```python
from build123d import *

# Parameters (mm, degrees)
SKETCH1_R           = 13.335
SKETCH1_R_2         = 8.255
SKETCH1_R_3         = 1.8288
BOSS_EXTRUDE1_DEPTH = 0.762
BOSS_EXTRUDE2_START = 1.524
SKETCH2_R           = 13.335
SKETCH2_R_2         = 12.573
BOSS_EXTRUDE2_DEPTH = 1.524


with BuildPart() as part:
    # Sketch1 → Boss-Extrude1 (new body)
    with BuildSketch(Plane.XY):
        with Locations(Location((0, 0, 0), (0, 0, 180))):
            Circle(SKETCH1_R)
        with Locations(Location((0, 0, 0), (0, 0, 180))):
            Circle(SKETCH1_R_2, mode=Mode.SUBTRACT)
        with Locations(Location((8.919971224, 5.542595082, 0), (0, 0, 180))):
            Circle(SKETCH1_R_3, mode=Mode.SUBTRACT)
        with Locations(Location((10.496219222, 0.340042532, 0), (0, 0, 180))):
            Circle(SKETCH1_R_3, mode=Mode.SUBTRACT)
        with Locations(Location((9.260013756, -4.95362414, 0), (0, 0, 180))):
            Circle(SKETCH1_R_3, mode=Mode.SUBTRACT)
        with Locations(Location((5.542595082, -8.919971224, 0), (0, 0, 180))):
            Circle(SKETCH1_R_3, mode=Mode.SUBTRACT)
        with Locations(Location((0.340042532, -10.496219222, 0), (0, 0, 180))):
            Circle(SKETCH1_R_3, mode=Mode.SUBTRACT)
        with Locations(Location((-4.95362414, -9.260013756, 0), (0, 0, 180))):
            Circle(SKETCH1_R_3, mode=Mode.SUBTRACT)
        with Locations(Location((-8.919971224, -5.542595082, 0), (0, 0, 180))):
            Circle(SKETCH1_R_3, mode=Mode.SUBTRACT)
        with Locations(Location((-10.496219222, -0.340042532, 0), (0, 0, 180))):
            Circle(SKETCH1_R_3, mode=Mode.SUBTRACT)
        with Locations(Location((-9.260013756, 4.95362414, 0), (0, 0, 180))):
            Circle(SKETCH1_R_3, mode=Mode.SUBTRACT)
        with Locations(Location((-5.542595082, 8.919971224, 0), (0, 0, 180))):
            Circle(SKETCH1_R_3, mode=Mode.SUBTRACT)
        with Locations(Location((-0.340042532, 10.496219222, 0), (0, 0, 180))):
            Circle(SKETCH1_R_3, mode=Mode.SUBTRACT)
        with Locations(Location((4.95362414, 9.260013756, 0), (0, 0, 180))):
            Circle(SKETCH1_R_3, mode=Mode.SUBTRACT)
    extrude(amount=BOSS_EXTRUDE1_DEPTH)

    # Sketch2 → Boss-Extrude2 (add)
    with BuildSketch(Plane(origin=(0, 0, 0), x_dir=(-1, 0, 0), z_dir=(0, 0, -1)).offset(BOSS_EXTRUDE2_START)):
        Circle(SKETCH2_R)
        with Locations(Location((0, 0, 0), (0, 0, 180))):
            Circle(SKETCH2_R_2, mode=Mode.SUBTRACT)
    extrude(amount=-BOSS_EXTRUDE2_DEPTH)


solid = part.part
```
Check sheet for the modelled part. Datum: model origin and axes. Units: mm. A direction names the side the tool comes from. Coordinates: 2 decimals unless noted, no trailing zeros. Write each loop counter-clockwise with the first axis right and the second up, starting at its lowest first coordinate (ties: lowest second). Pieces come first, ordered by that corner, then holes. Notation, with made-up numbers: (26.5, 27.25) -> (65.5, 27.25) arc R12 ccw to (65.5, 35.25) -> close; hole circle Ø1 at (-17.75, 32). An arc over 180 degrees is marked (long way). Use a Markdown table: item, result.
1. Sectioned sample at A-A (x = 0). Enter the section's corners in (y, z) (3 decimals).
Reported:
| item | result |
|---|---|
| outline | (-13.335, -1.524) -> (-12.573, -1.524) -> (-12.573, 0) -> (-12.293, 0) -> (-12.293, 0.762) -> (-13.335, 0.762) -> close; (-8.699, 0) -> (-8.255, 0) -> (-8.255, 0.762) -> (-8.699, 0.762) -> close; (8.255, 0) -> (8.699, 0) -> (8.699, 0.762) -> (8.255, 0.762) -> close; (12.293, 0) -> (12.573, 0) -> (12.573, -1.524) -> (13.335, -1.524) -> (13.335, 0.762) -> (12.293, 0.762) -> close |
2. Scan lines: line 1 along Y through (x, z) = (-1, 0.5); line 2 along Y through (x, z) = (0, -0.75) (3 decimals); line 3 along Y through (x, z) = (9.25, 0.1). Record each from-to range of solid material in increasing order.
Reported:
| item | result |
|---|---|
| line 1 | y = -13.3 to -11.74, -9.25 to -8.19, 8.19 to 8.79, 12.2 to 13.3 |
| line 2 | y = -13.335 to -12.573, 12.573 to 13.335 |
| line 3 | y = -9.61 to -6.78, -3.12 to -1, 1.68 to 3.74, 7.34 to 9.61 |
3. Release check for a two-part mould opening along X. For faces 1 (the flat face through (9, 9, -1.524)), 2 (the cylindrical face through (-7.572, -6.779, 0.376)), 3 (the cylindrical face through (1.74, 13.22, -0.4)) record: pulls with the +X half, pulls with the -X half, needs draft (parallel to the pull), parting line crosses it, or undercut.
Reported:
| item | result |
|---|---|
| face 1 | needs draft |
| face 2 | undercut |
| face 3 | parting line crosses it |
4. Sectioned sample at C-C (z = 0.45). Give the number of separate pieces and of enclosed holes in the cut face, plus the area to 3 significant figures.
Reported:
| item | result |
|---|---|
| separate pieces | 1 |
| enclosed holes | 13 |
| area | 218 mm2 |
5. Tool access check on faces 4 (the cylindrical face through (0.74, -8.71, 0.38)), 5 (the flat face through (3.8, -7.5, 0)). Record the directions out of +Z, -Z, +X, -X, +Y, -Y that give a thin tool (end or side, any length) a straight path to the whole face; none if there is none.
Reported:
| item | result |
|---|---|
| face 4 | +Z, -Z |
| face 5 | -Z |
6. Go/stop test with flat-tipped pins: pin 1 Ø1 at (x, z) = (2.5, -1.5) entering from -Y; pin 2 Ø1 at (x, z) = (-7.5, -1) entering from -Y; pin 3 Ø4 at (x, y) = (9.26, -4.95) entering from -Z. Record where each tip stops, or that it passes through.
Reported:
| item | result |
|---|---|
| pin 1 | stops at y = -13.18 |
| pin 2 | stops at y = -11.35 |
| pin 3 | stops at z = 0 |
7. Sectioned sample at D-D (z = -1.2). Enter the section's corners in (x, y) (3 decimals), plus the area to 3 significant figures.
Reported:
| item | result |
|---|---|
| outline | circle Ø26.67 at (0, 0); hole circle Ø25.146 at (0, 0) |
| area | 62.0 mm2 |
